Can you work these out from the model? Positions are in its coordinate system, mm. A direction names the side the tool comes from. Give positions to 0.01 mm unless a question says otherwise; leave off trailing zeros. Loops run counter-clockwise (first coordinate to the right, second up) from the corner with the lowest first, then second, coordinate; pieces in that order, holes last.
from build123d import *

# Parameters (mm, degrees)
F0_W     = 139.073908329
F0_H     = 85.957378149
F0_W_2   = 116.2280887365
F0_H_2   = 62.5404193997
F1_DEPTH = 63.5
F2_W     = 51.4795817435
F2_H     = 101.4539152384
F3_DEPTH = 25.4
F4_DEPTH = 25.4
F5_R     = 9.7930895965
F6_DEPTH = 69.5379541645


# Not quite as in the source:
# - a pattern or mirror of a feature is missing from the dataset's text; its kind, count and spacing are read off the source's solid


with BuildPart() as f1:
    # F0 (on Top) → F1 (new body)
    with BuildSketch(Plane.XY):
        Rectangle(F0_W, F0_H)
        Rectangle(F0_W_2, F0_H_2, mode=Mode.SUBTRACT)
    extrude(amount=F1_DEPTH)

    # F2 (on Top) → F3 (join)
    with BuildSketch(Plane.XY):
        Rectangle(F2_W, F2_H)
    extrude(amount=F3_DEPTH)

    # F2 (on Top) → F4 (cut)
    with BuildSketch(Plane.XY):
        Rectangle(F2_W, F2_H)
    extrude(amount=F4_DEPTH, mode=Mode.SUBTRACT)

    # F5 (on Right) → F6 (cut, through all)
    with BuildSketch(Plane.YZ):
        with Locations((0, 36.6961322725)):
            Circle(F5_R)
    f6 = extrude(amount=-F6_DEPTH, mode=Mode.SUBTRACT)

    # F6_copies: F6 across plane
    add(f6.mirror(Plane(origin=(0, 0, 0), x_dir=(0, 0, 1), z_dir=(1, 0, 0))), mode=Mode.SUBTRACT)


solid = f1.part
(1) Suppose I cut it at C-C on z = 19. List the corners of the cut face in (x, y) for me, plus the area to 3 significant figures.
Returned:
outline: (-69.54, -42.98) - (-25.74, -42.98) - (-25.74, -31.27) - (-58.11, -31.27) - (-58.11, 31.27) - (-25.74, 31.27) - (-25.74, 42.98) - (-69.54, 42.98) - close; (25.74, -42.98) - (69.54, -42.98) - (69.54, 42.98) - (25.74, 42.98) - (25.74, 31.27) - (58.11, 31.27) - (58.11, -31.27) - (25.74, -31.27) - close
area: 3,480 mm2
(2) Suppose I cut it at D-D on y = -28. List the corners of the cut face in (x, z) for me, plus the area to 3 significant figures.
Returned:
outline: (-69.54, 0) - (-58.11, 0) - (-58.11, 63.5) - (-69.54, 63.5) - close; (58.11, 0) - (69.54, 0) - (69.54, 63.5) - (58.11, 63.5) - close
area: 1,450 mm2
(3) Suppose I cut it at B-B on x = -54.5. List the corners of the cut face in (y, z) for me, plus the area to 3 significant figures.
Returned:
outline: (-42.98, 0) - (-31.27, 0) - (-31.27, 63.5) - (-42.98, 63.5) - close; (31.27, 0) - (42.98, 0) - (42.98, 63.5) - (31.27, 63.5) - close
area: 1,490 mm2
(4) Please list where these lines run through material, in increasing order: probe 1 along X at (y, z) = (-19.5, 51); probe 2 along Y at (x, z) = (35, 12); probe 3 along Z at (x, y) = (-61.5, 0).
Returned:
probe 1: x = -69.54 to -58.11, 58.11 to 69.54
probe 2: y = -42.98 to -31.27, 31.27 to 42.98
probe 3: z = 0 to 26.9, 46.49 to 63.5
(5) Thinking about a two-plate mould opening in X: for faces 4 (the flat face through (-69.537, -1, 24)), 5 (the flat face through (-63, 1, 0)), 6 (the flat face through (69.537, -1, 24)), 7 (the flat face through (58.114, 0, 24)), which applies, pulls with the +X half, pulls with the -X half, needs draft (parallel to the pull), parting line crosses it, or undercut?
Returned:
face 4: pulls with the -X half
face 5: needs draft
face 6: pulls with the +X half
face 7: undercut
(6) Will this pin go through, and if not, where does the flat tip stop? P1, Ø13, axis at x = -11.5, y = -39, coming from the -Z side.
Returned:
P1: stops at z = 25.4
(7) Which directions (+Z, -Z, +X, -X, +Y, -Y) give clear straight access to the entire face, cutting with the end or side of a thin tool? Please do faces 1 (the flat face through (-1, -31.27, 38)), 2 (the flat face through (-1, -42.979, 31)), 3 (the flat face through (25.74, 37, 13)).
Returned:
face 1: +Z, -Z
face 2: +Z, -Z, +X, -X, -Y
face 3: -Z, +Y, -Y
(8) Suppose I cut it at A-A on y = 0. List the corners of the cut face in (x, z) for me.
Returned:
outline: (-69.54, 0) - (-58.11, 0) - (-58.11, 26.9) - (-69.54, 26.9) - close; (-69.54, 46.49) - (-58.11, 46.49) - (-58.11, 63.5) - (-69.54, 63.5) - close; (58.11, 0) - (69.54, 0) - (69.54, 26.9) - (58.11, 26.9) - close; (58.11, 46.49) - (69.54, 46.49) - (69.54, 63.5) - (58.11, 63.5) - close
